Autodesk Inventor part; units mm, degrees
ref_plane "YZ Plane" through (0, 0, 0) normal (1, 0, 0) x (0, 1, 0)
ref_plane "XZ Plane" through (0, 0, 0) normal (0, 1, 0) x (-1, 0, 0)
ref_plane "XY Plane" through (0, 0, 0) normal (0, 0, 1) x (1, 0, 0)
sketch "Sketch1" plane through (0, 0, 0) normal (1, 0, 0) x (0, 1, 0)
  line L0 (1.0612, -13.162) -> (11.0434, 4.1278)
  line L1 (-1.0612, 13.162) -> (-11.0434, -4.1278)
  line L2 (6.0523, -4.5171) -> (-6.0523, 4.5171) construction
  line L3 (-26.5933, 0) -> (26.5933, 0) construction
  line L4 (0, -35.5609) -> (0, 35.5609) construction
  line L5 (11.0434, 4.1278) -> (18.9952, 17.9006)
  line L6 (18.9952, 17.9006) -> (6.0048, 25.4006)
  line L7 (-1.0612, 13.162) -> (6.0048, 25.4006)
  line L8 (1.0612, -13.162) -> (-6.0048, -25.4006)
  line L9 (-6.0048, -25.4006) -> (-18.9952, -17.9006)
  line L10 (-18.9952, -17.9006) -> (-11.0434, -4.1278)
  point P0 (0, 0)
  dimension "d1" = 15
  dimension "d2" = 50
  dimension "d4" = 60
extrude "Extrusion1" add sketch "Sketch1" along normal blind 6
sketch "Sketch2" plane through (0, 0, 0) normal (-1, 0, 0) x (0, 0, 1)
  point P0 (0, 0)
hole "Hole1" at (0, 0, 0) direction (1, 0, 0) diameter 8 end through all
sketch "Sketch3" plane through (0, 0, 0) normal (0, 1, 0) x (-1, 0, 0)
  line L0 (-6, -25.4006) -> (-6, 17.9006) construction
  line L1 (0, -25.4006) -> (0, 17.9006) construction
  line L2 (1.2, 0) -> (-7.2, 0) construction
  line L3 (0, 0) -> (-6, 0) construction
  point P0 (-6, -17.5083)
  point P1 (-6, 5.0083)
  point P2 (0, 5.0083)
  point P3 (0, -17.5083)
  point P4 (-3, 0)
  point P5 (-3, 0)
hole "Hole2" at (3, 0, 0) direction (0, -1, 0) diameter 3.242 end through all
sketch "Sketch4" plane through (0, 0, 0) normal (-1, 0, 0) x (0, 0, 1)
  circle A0 centre (0, 0) radius 4 construction
  line L0 (-25.4006, -6.0048) -> (17.9006, 18.9952) construction
  line L1 (25.4006, 6.0048) -> (-17.9006, -18.9952) construction
  line L2 (-26.825, -15.4874) -> (32.6029, 18.8233) construction
  line L3 (7.5083, 12.9952) -> (-15.0083, -0.0048) construction
  line L4 (-17.9006, -18.9952) -> (-25.4006, -6.0048)
  line L5 (17.9006, 18.9952) -> (25.4006, 6.0048)
  point P0 (5.0083, 17.3253)
  point P1 (-17.5083, 4.3253)
  point P2 (17.3205, 10)
  point P3 (-17.3205, -10)
  dimension "d21" = 20
  dimension "d22" = 20
hole "Hole3" at (0, 10, 17.3205) at (0, -10, -17.3205) direction (1, 0, 0) diameter 3.459 depth 4 tip angle 118
fillet "Fillet1" radius 6 4 edges at (3, 18.9952, 17.9006) (3, 6.0048, 25.4006) (3, -6.0048, -25.4006) (3, -18.9952, -17.9006)
The listing builds one solid part. Answer for the finished solid, in the listing's coordinates (mm). A direction names the side the tool comes from. Round coordinates to 2 decimals unless told otherwise and drop trailing zeros. Loops run counter-clockwise (first coordinate to the right, second up) from the corner with the lowest first, then second, coordinate; pieces in that order, holes last. Notation, with made-up numbers: (28.5, -22) - (62.5, -22) arc R25 ccw to (62.5, 12) - close; hole circle Ø9 at (79, -11). An arc over 180 degrees is marked (long way). Use one line per item in the form item = value. Start each with the question number.
1. The part is cut by section B-B on z = 0. Determine the outline of the cut face in (x, y).
2. A tool of negligible diameter and unlimited length cuts with its end or side. For faces 1 (the face through (2.028, 9.924, 15.593)), 2 (the face through (3.042, 16.611, 17.194)), from which of +Z, -Z, +X, -X, +Y, -Y can it reach the whole face along a straight path? Write none if from no direction.
3. The part is cut by section C-C on x = 0.75. Determine the outline of the cut face in (y, z), then the cut area to 3 significant figures.
4. The part is cut by section D-D on y = 7. Determine the outline of the cut face in (x, z), then the cut area to 3 significant figures.
5. The part is cut by section A-A on y = 0. Determine the outline of the cut face in (x, z).
6. Given pin 1 Ø7 at (y, z) = (0, 0) entering from -X; pin 2 Ø2 at (x, y) = (3.5, 5.5) entering from +Z; pin 3 Ø1 at (x, y) = (0.5, -11) entering from +Z; pin 4 Ø1.5 at (x, z) = (2, 11) entering from +Y, each flat-ended and moving along its own axis, determine where each tip first touches the part or whether it passes through.
7. For a pull along X with two mould halves and no side action, classify faces 3 (the face through (2.96, -12.48, -21.66)), 4 (the face through (2.93, -6.01, -1.62)), 5 (the face through (4.86, -9.99, -17.62)) as pulls with the +X half, pulls with the -X half, needs draft (parallel to the pull), parting line crosses it, or undercut.
8. Consider line 1 (Z direction, x = 3, y = -7.5); line 2 (Z direction, x = 3, y = -8.15); line 3 (X direction, y = -7, z = -1). Determine where each line is inside the solid, lowest interval first. Write a range as [from, to].
Geometry check:
q1.outline = (0, -8.66) - (1.38, -8.66) - (1.38, -4) - (0, -4) - close; (0, 4) - (6, 4) - (6, 8.66) - (0, 8.66) - close; (4.62, -8.66) - (6, -8.66) - (6, -4) - (4.62, -4) - close
q2.face_1 = -X
q2.face_2 = +X, -X, +Y
q3.outline = (-16, -12.7) arc R6 ccw to (-13.8, -20.9) - (-11.2, -22.4) arc R6 ccw to (-3, -20.2) - (1.06, -13.16) - (11.04, 4.13) - (16, 12.7) arc R6 ccw to (13.8, 20.9) - (11.2, 22.4) arc R6 ccw to (3, 20.2) - (-1.06, 13.16) - (-11.04, -4.13) - close; hole circle Ø3.46 at (-10, -17.32); hole circle Ø8 at (0, 0); hole circle Ø3.46 at (10, 17.32)
q3.area = 650 mm^2
q4.outline = (0, -2.88) - (6, -2.88) - (6, 23.08) - (0, 23.08) - close
q4.area = 156 mm^2
q5.outline = (0, -15) - (6, -15) - (6, -4) - (0, -4) - close; (0, 4) - (6, 4) - (6, 15) - (0, 15) - close
q6.pin_1 = through
q6.pin_2 = 22.96
q6.pin_3 = -3.19
q6.pin_4 = 15.44
q7.face_3 = needs draft
q7.face_4 = undercut
q7.face_5 = pulls with the -X half
q8.line_1 = [-23.16, -1.62], [1.62, 2.01]
q8.line_2 = [-23.2, -1.62]
q8.line_3 = [0, 1.72], [4.28, 6]
